The listing builds one solid part. Answer for the finished solid, in the listing's coordinates (mm). A direction names the side the tool comes from. Round coordinates to 2 decimals unless told otherwise and drop trailing zeros. Write each loop counter-clockwise with the first axis right and the second up, starting at its lowest first coordinate (ties: lowest second). Pieces come first, ordered by that corner, then holes. Notation, with made-up numbers: (21.25, 30.25) - (76.25, 30.25) arc R21 ccw to (76.25, 37.25) - close; hole circle Ø2 at (-16.75, 2). An arc over 180 degrees is marked (long way). Use a Markdown table: item, result. Add a question column.
1) A cutting plane is placed at A-A (z = 16). Give the vertices of the cut face in (x, y), then the cut area to 3 significant figures.
2) Each of these flat-tipped pins is pushed along its axis until it touches: P1, Ø2.5, axis at y = 11, z = 20.7, coming from the -X side; P2, Ø0.8, axis at x = 21, z = 24.5, coming from the +Y side; P3, Ø7, axis at y = 10.5, z = 8, coming from the -X side. Where does it stop, or does it pass through?
3) A cutting plane is placed at B-B (z = 20.7). State how many separate pieces and enclosed holes the cut face has, then the cut area to 3 significant figures.
4) A tool of negligible diameter and unlimited length cuts with its end or side. For faces 5 (the flat face through (17.25, 9, 19)), 6 (the flat face through (3.5, 12, 9)), 7 (the flat face through (10.09, 16.79, 10.87)), from which of +Z, -Z, +X, -X, +Y, -Y can it reach the whole face along a straight path? Write none if from no direction.
5) Determine the mould class of faces 1 (the flat face through (9.9, 18.3, 9.56)), 2 (the flat face through (20.874, 4.212, 20.404)), 3 (the flat face through (10, 2, 0)), 4 (the flat face through (-0.5, 6, 12)) for opening direction Y: +Y half, -Y half, draft (parallel to the pull), parting line (faces both ways), or undercut.
6) Find the intervals of material crossed by probe 1 along Y at (x, z) = (17.9, 20.7); probe 2 along X at (y, z) = (14, 12); probe 3 along X at (y, z) = (2.25, 13), in increasing order. Write a range as from..to.
7) A cutting plane is placed at C-C (x = 9.25). Give the vertices of the cut face in (y, z), then the cut area to 3 significant figures.
```python
from build123d import *

# Parameters (mm, degrees)
SKIZZE1_W                             = 20
SKIZZE1_H                             = 22
AUFSATZ_LINEAR_AUSTRAGEN1_DEPTH       = 35
SKIZZE2_R                             = 5.5
SCHNITT_LINEAR_AUSTRAGEN1_DEPTH       = 11
SKIZZE3_R                             = 6.25
SCHNITT_LINEAR_AUSTRAGEN2_DEPTH       = 8
SKIZZE5_W                             = 14.5
SKIZZE5_H                             = 18.25
SCHNITT_LINEAR_AUSTRAGEN3_DEPTH       = 9
SKIZZE13_W                            = 20
SKIZZE13_H                            = 11
SCHNITT_LINEAR_AUSTRAGEN6_DEPTH       = 18
SCHNITT_LINEAR_AUSTRAGEN7_DEPTH       = 46.923850013
VERRUNDUNG1_R                         = 0.5
FASE1_SIZE                            = 3
FASE2_SIZE                            = 3
FASE3_SIZE                            = 3
FASE4_SIZE                            = 1.5
SKIZZE17_W                            = 6
SKIZZE17_H                            = 3.5
SCHNITT_LINEAR_AUSTRAGEN8_DEPTH       = 45.25
SCHNITT_LINEAR_AUSTRAGEN9_REACH       = 47.924
SKIZZE18_W                            = 3.75
SKIZZE18_H                            = 11
SCHNITT_LINEAR_AUSTRAGEN10_DEPTH      = 6.5
SCHNITT_LINEAR_AUSTRAGEN10_DEPTH_BACK = 6.5
AUFSATZ_LINEAR_AUSTRAGEN2_DEPTH       = 24
SCHNITT_LINEAR_AUSTRAGEN11_DEPTH      = 22
SKIZZE26_W                            = 5.75
SKIZZE26_H                            = 1
SCHNITT_LINEAR_AUSTRAGEN12_DEPTH      = 4
AUFSATZ_LINEAR_AUSTRAGEN3_DEPTH       = 14.25
SKIZZE28_W                            = 2.25
SKIZZE28_H                            = 3
AUFSATZ_LINEAR_AUSTRAGEN4_DEPTH       = 7
AUFSATZ_LINEAR_AUSTRAGEN6_DEPTH       = 2.25
SCHNITT_LINEAR_AUSTRAGEN13_REACH      = 47.128
SKIZZE32_R                            = 1
SCHNITT_LINEAR_START                  = 10
SKIZZE33_R                            = 1.9
SCHNITT_LINEAR_AUSTRAGEN14_DEPTH      = 1.5
SKIZZE34_R                            = 1.9
SCHNITT_LINEAR_AUSTRAGEN15_DEPTH      = 1.5


with BuildPart() as part:
    # Skizze1 → Aufsatz-Linear austragen1 (new body)
    with BuildSketch(Plane.XY):
        with Locations((10, 11)):
            Rectangle(SKIZZE1_W, SKIZZE1_H)
    extrude(amount=AUFSATZ_LINEAR_AUSTRAGEN1_DEPTH)

    # Skizze2 → Schnitt-Linear austragen1 (cut)
    with BuildSketch(Plane.XY.offset(35)):
        with Locations((10, 11)):
            Circle(SKIZZE2_R)
    extrude(amount=-SCHNITT_LINEAR_AUSTRAGEN1_DEPTH, mode=Mode.SUBTRACT)

    # Skizze3 → Schnitt-Linear austragen2 (cut)
    with BuildSketch(Plane.XY.offset(35)):
        with Locations((10, 11)):
            Circle(SKIZZE3_R)
    extrude(amount=-SCHNITT_LINEAR_AUSTRAGEN2_DEPTH, mode=Mode.SUBTRACT)

    # Skizze5 → Schnitt-Linear austragen3 (cut)
    with BuildSketch(Plane.XY.offset(24)):
        with Locations((10, 12.875)):
            Rectangle(SKIZZE5_W, SKIZZE5_H)
    extrude(amount=-SCHNITT_LINEAR_AUSTRAGEN3_DEPTH, mode=Mode.SUBTRACT)

    # Skizze13 → Schnitt-Linear austragen6 (cut)
    with BuildSketch(Plane.XY.offset(35)):
        with Locations((10, 16.5)):
            Rectangle(SKIZZE13_W, SKIZZE13_H)
    extrude(amount=-SCHNITT_LINEAR_AUSTRAGEN6_DEPTH, mode=Mode.SUBTRACT)

    # Skizze16 → Schnitt-Linear austragen7 (cut, through all)
    with BuildSketch(Plane.ZY):
        Polygon((14, 22), (5, 14.5), (0, 4), (0, 22), align=None)
    extrude(amount=-SCHNITT_LINEAR_AUSTRAGEN7_DEPTH, mode=Mode.SUBTRACT)

    # Verrundung1
    verrundung1_edges = [part.edges().sort_by_distance(p)[0] for p in [
        (17.25, 11, 20.5),
        (3.75, 11, 31),
        (2.75, 11, 20.5),
        (4.5, 11, 25.5),
        (16.25, 11, 31),
        (15.5, 11, 25.5),
    ]]
    fillet(verrundung1_edges, radius=VERRUNDUNG1_R)

    # Fase1
    fase1_edges = [part.edges().sort_by_distance(p)[0] for p in [
        (20, 22, 15.5),
        (0, 22, 15.5),
    ]]
    chamfer(fase1_edges, length=FASE1_SIZE)

    # Fase2
    fase2_edges = [part.edges().sort_by_distance(p)[0] for p in [
        (0, 16.75, 7.7),
        (20, 16.75, 7.7),
    ]]
    chamfer(fase2_edges, length=FASE2_SIZE)

    # Fase3
    fase3_edges = [part.edges().sort_by_distance(p)[0] for p in [
        (20, 6.012857042, 0.958503353),
        (20, 2, 0),
        (0, 6.012857042, 0.958503353),
        (0, 2, 0),
    ]]
    chamfer(fase3_edges, length=FASE3_SIZE)

    # Fase4
    fase4_edges = [part.edges().sort_by_distance(p)[0] for p in [
        (20, 11, 26),
        (0, 11, 26),
    ]]
    chamfer(fase4_edges, length=FASE4_SIZE)

    # Skizze17 → Schnitt-Linear austragen8 (cut, through all)
    with BuildSketch(Plane(origin=(0, 3.75, 0), x_dir=(1, 0, 0), z_dir=(0, 1, 0))):
        with Locations((5.75, -16.75)):
            Rectangle(SKIZZE17_W, SKIZZE17_H)
    extrude(amount=-SCHNITT_LINEAR_AUSTRAGEN8_DEPTH, mode=Mode.SUBTRACT)

    # Schnitt-Linear austragen9: up to this face of the body (flat: up to its plane)
    schnitt_linear_austragen9_end = Plane(part.part.faces().sort_by_distance((20, 6.280299508, 18.20769637))[0])
    # Skizze18 → Schnitt-Linear austragen9 (cut, up to the picked face)
    with BuildSketch(Plane.ZY, mode=Mode.PRIVATE) as schnitt_linear_austragen9_sk1:
        with Locations((33.125, 5.5)):
            Rectangle(SKIZZE18_W, SKIZZE18_H)
    schnitt_linear_austragen9_tool1 = split(extrude(schnitt_linear_austragen9_sk1.sketch, amount=-SCHNITT_LINEAR_AUSTRAGEN9_REACH, mode=Mode.PRIVATE), bisect_by=schnitt_linear_austragen9_end, keep=Keep.BOTH, mode=Mode.PRIVATE)
    add(schnitt_linear_austragen9_tool1.solids().sort_by(Axis((0, 5.5, 33.125), (1, 0, 0)))[0], mode=Mode.SUBTRACT)

    # Skizze22 → Schnitt-Linear austragen10 (cut, two sides)
    with BuildSketch(Plane.ZY.offset(-10)) as schnitt_linear_austragen10_sk:
        Polygon((15, 20.229916775), (6.617209038, 13.24425764), (5.760028677, 11.896060222), (3.760028677, 11.896060222), (0.88063989, 5.849343769), (6.035195751, 5.849343769), (15, 5.849343769), align=None)
    extrude(amount=SCHNITT_LINEAR_AUSTRAGEN10_DEPTH, mode=Mode.SUBTRACT)
    extrude(schnitt_linear_austragen10_sk.sketch, amount=-SCHNITT_LINEAR_AUSTRAGEN10_DEPTH_BACK, mode=Mode.SUBTRACT)

    # Skizze23 → Aufsatz-Linear austragen2 (add)
    with BuildSketch(Plane.XY.offset(31.25)):
        Polygon((0, 8.353013166), (-4, 0), (0, 0), align=None)
    aufsatz_linear_austragen2 = extrude(amount=-AUFSATZ_LINEAR_AUSTRAGEN2_DEPTH)

    # Spiegeln1: Aufsatz-Linear austragen2 across plane
    add(aufsatz_linear_austragen2.mirror(Plane.ZY.offset(-10)))

    # Skizze24 → Schnitt-Linear austragen11 (cut)
    with BuildSketch(Plane.XY.offset(31.25)):
        Polygon((0.460828855, 1.5), (-2.172951263, 1.5), (0.460828855, 7), align=None)
    schnitt_linear_austragen11 = extrude(amount=-SCHNITT_LINEAR_AUSTRAGEN11_DEPTH, mode=Mode.SUBTRACT)

    # Skizze26 → Schnitt-Linear austragen12 (cut)
    with BuildSketch(Plane.ZY.offset(-16.5)):
        with Locations((12.125, 6.349343769)):
            Rectangle(SKIZZE26_W, SKIZZE26_H)
    schnitt_linear_austragen12 = extrude(amount=-SCHNITT_LINEAR_AUSTRAGEN12_DEPTH, mode=Mode.SUBTRACT)

    # Spiegeln2: Schnitt-Linear austragen12 across plane
    add(schnitt_linear_austragen12.mirror(Plane.ZY.offset(-10)), mode=Mode.SUBTRACT)

    # Spiegeln3: Schnitt-Linear austragen11 across plane
    add(schnitt_linear_austragen11.mirror(Plane.ZY.offset(-10)), mode=Mode.SUBTRACT)

    # Skizze27 → Aufsatz-Linear austragen3 (add)
    with BuildSketch(Plane.XY.offset(17)):
        Polygon((0, 9.5), (1.5, 11), (0, 11), align=None)
    aufsatz_linear_austragen3 = extrude(amount=AUFSATZ_LINEAR_AUSTRAGEN3_DEPTH)

    # Spiegeln4: Aufsatz-Linear austragen3 across plane
    add(aufsatz_linear_austragen3.mirror(Plane.ZY.offset(-10)))

    # Skizze28 → Aufsatz-Linear austragen4 (add)
    with BuildSketch(Plane.XY.offset(17)):
        with Locations((1.125, 12.5)):
            Rectangle(SKIZZE28_W, SKIZZE28_H)
    aufsatz_linear_austragen4 = extrude(amount=AUFSATZ_LINEAR_AUSTRAGEN4_DEPTH)

    # Skizze31 → Aufsatz-Linear austragen6 (add)
    with BuildSketch(Plane.ZY):
        Polygon((24, 14), (26, 11), (24, 11), align=None)
    aufsatz_linear_austragen6 = extrude(amount=-AUFSATZ_LINEAR_AUSTRAGEN6_DEPTH)

    # Schnitt-Linear austragen13: up to this face of the body (flat: up to its plane)
    schnitt_linear_austragen13_end = Plane(part.part.faces().sort_by_distance((2.75, 8.51118677, 18.308365759))[0])
    # Skizze32 → Schnitt-Linear austragen13 (cut, up to the picked face)
    with BuildSketch(Plane.ZY, mode=Mode.PRIVATE) as schnitt_linear_austragen13_sk1:
        with Locations((20.7, 11)):
            Circle(SKIZZE32_R)
    schnitt_linear_austragen13_tool1 = split(extrude(schnitt_linear_austragen13_sk1.sketch, amount=-SCHNITT_LINEAR_AUSTRAGEN13_REACH, mode=Mode.PRIVATE), bisect_by=schnitt_linear_austragen13_end, keep=Keep.BOTH, mode=Mode.PRIVATE)
    schnitt_linear_austragen13 = schnitt_linear_austragen13_tool1.solids().sort_by(Axis((0, 11, 20.7), (1, 0, 0)))[0]
    add(schnitt_linear_austragen13, mode=Mode.SUBTRACT)

    # Skizze33 → Schnitt-Linear austragen14 (cut)
    with BuildSketch(Plane.ZY.offset(-10).offset(SCHNITT_LINEAR_START)):
        with Locations(Location((20.7, 11, 0), (0, 0, 180))):
            Circle(SKIZZE33_R)
    extrude(amount=-SCHNITT_LINEAR_AUSTRAGEN14_DEPTH, mode=Mode.SUBTRACT)

    # Spiegeln6: Aufsatz-Linear austragen4, Aufsatz-Linear austragen6 across plane
    add(aufsatz_linear_austragen4.mirror(Plane.ZY.offset(-10)))
    add(aufsatz_linear_austragen6.mirror(Plane.ZY.offset(-10)))

    # Spiegeln8: Schnitt-Linear austragen13 across plane
    add(schnitt_linear_austragen13.mirror(Plane.ZY.offset(-10)), mode=Mode.SUBTRACT)

    # Skizze34 → Schnitt-Linear austragen15 (cut)
    with BuildSketch(Plane(origin=(20, 0, 0), x_dir=(0, 0, -1), z_dir=(1, 0, 0))):
        with Locations((-20.7, 11)):
            Circle(SKIZZE34_R)
    extrude(amount=-SCHNITT_LINEAR_AUSTRAGEN15_DEPTH, mode=Mode.SUBTRACT)


solid = part.part
```
Entries:
| question | item | result |
|---|---|---|
| 1 | outline | (-4, 0) - (2.75, 0) - (2.75, 21.75) - (0, 19) - (0, 8.35) - close; (8.75, 0) - (24, 0) - (20, 8.35) - (20, 19) - (17.25, 21.75) - (17.25, 3.75) - (8.75, 3.75) - close; hole (-2.17, 1.5) - (0.46, 1.5) - (0.46, 7) - close; hole (19.54, 1.5) - (22.17, 1.5) - (19.54, 7) - close |
| 1 | area | 163 mm² |
| 2 | P1 | stops at x = 1.5 |
| 2 | P2 | stops at y = 7.1 |
| 2 | P3 | stops at x = -0.65 |
| 3 | separate pieces | 3 |
| 3 | enclosed holes | 2 |
| 3 | area | 132 mm² |
| 4 | face 5 | +Y |
| 4 | face 6 | none |
| 4 | face 7 | +Z |
| 5 | face 1 | +Y half |
| 5 | face 2 | undercut |
| 5 | face 3 | draft |
| 5 | face 4 | undercut |
| 6 | probe 1 | y = 0..10, 12..14 |
| 6 | probe 2 | x = 0..3.5, 16.5..20 |
| 6 | probe 3 | x = -2.92..-1.81, 0.46..19.54, 21.81..22.92 |
| 7 | outline | (0, 0) - (4, 0) - (5.85, 0.88) - (5.85, 15) - (3.75, 15) - (3.75, 24) - (5.55, 24) - (5.55, 27) - (4.8, 27) - (4.8, 31.25) - (0, 31.25) - close; (11.9, 3.76) - (14.5, 5) - (22, 14) - (22, 15) - (20.23, 15) - (13.24, 6.62) - (11.9, 5.76) - close |
| 7 | area | 185 mm² |
